Read the model definition and answer for the solid it produces. Units are mm, in the model's axes. Round coordinates to 2 decimals unless told otherwise and drop trailing zeros. Order: outer loops, then holes, each group sorted by start corner. A loop starts at its lowest first (then second) coordinate and runs counter-clockwise, first axis right, second up. Notation, with made-up numbers: (-20.75, -39.5) - (34.25, -39.5) arc R19 ccw to (34.25, -14.5) - close; hole circle Ø8 at (-32.75, -28). An arc over 180 degrees is marked (long way). Put each result on its own line as item: value. Start each with the question number.
Q1. Section A-A on x = 0 is taken. Give the vertices of the cut face in (y, z), then the cut area to 3 significant figures.
Q2. Find the intervals of material crossed by line 1 along Y through (x, z) = (1.5, 16.5); line 2 along Y through (x, z) = (-4.5, -22); line 3 along X through (y, z) = (39.5, 19.5), in increasing order. Write a range as from..to.
Q3. Section B-B on z = 0 is taken. Give the vertices of the cut face in (x, y), then the cut area to 3 significant figures.
Q4. Each of these flat-tipped pins is pushed along its axis until it touches: pin 1 Ø10 at (x, y) = (18, 29) entering from -Z; pin 2 Ø1 at (x, y) = (12.5, 50) entering from -Z; pin 3 Ø3 at (y, z) = (28.5, 9.5) entering from +X. Where does it stop, or does it pass through?
Q5. Section C-C on y = 14.5 is taken. Give the vertices of the cut face in (x, z).
Q6. For a pull along Y with two mould halves and no side action, classify faces 1 (the face through (4.01, 54.34, -18.04)), 2 (the face through (0, 0, 0)), 3 (the face through (14.59, 66.04, -11.19)), 4 (the face through (0, 71, 0)) as pulls with the +Y half, pulls with the -Y half, needs draft (parallel to the pull), parting line crosses it, or undercut.
Q7. Section D-D on y = 59 is taken. Give the vertices of the cut face in (x, z), then the cut area to 3 significant figures.
from build123d import *

# Parameters (mm, degrees)
SKETCH1_R           = 25.05
BOSS_EXTRUDE1_DEPTH = 71


with BuildPart() as part:
    # Sketch1 → Boss-Extrude1 (new body)
    with BuildSketch(Plane(origin=(0, 0, 0), x_dir=(1, 0, 0), z_dir=(0, 1, 0))):
        Circle(SKETCH1_R)
    extrude(amount=BOSS_EXTRUDE1_DEPTH)

    # Sketch2 → Cut-Revolve1 (revolve, cut)
    with BuildSketch(Plane.XY):
        with BuildLine():
            Line((-25.05, 67.7), (-18.045116148, 65.953486299))
            ThreePointArc((-18.045116148, 65.953486299), (-13.55, 60.2), (-18.045116148, 54.446513701))
            Line((-18.045116148, 54.446513701), (-25.05, 52.7))
            Line((-25.05, 52.7), (-25.05, 67.7))
        make_face()
    revolve(axis=Axis((0, -3.55, 0), (0, 1, 0)), mode=Mode.SUBTRACT)


solid = part.part
Findings:
1. outline: (0, -25.05) - (52.7, -25.05) - (54.45, -18.05) arc R5.93 cw to (65.95, -18.05) - (67.7, -25.05) - (71, -25.05) - (71, 25.05) - (67.7, 25.05) - (65.95, 18.05) arc R5.93 cw to (54.45, 18.05) - (52.7, 25.05) - (0, 25.05) - close
1. area: 3,290 mm2
2. line 1: 0..55.03, 65.37..71
2. line 2: 0..53.35, 67.05..71
2. line 3: -15.72..15.72
3. outline: (-25.05, 0) - (25.05, 0) - (25.05, 52.7) - (18.05, 54.45) arc R5.93 cw to (18.05, 65.95) - (25.05, 67.7) - (25.05, 71) - (-25.05, 71) - (-25.05, 67.7) - (-18.05, 65.95) arc R5.93 cw to (-18.05, 54.45) - (-25.05, 52.7) - close
3. area: 3,290 mm2
4. pin 1: z = -21.41
4. pin 2: z = -21.99
4. pin 3: x = 23.74
5. outline: circle Ø50.1 at (0, 0)
6. face 1: undercut
6. face 2: pulls with the -Y half
6. face 3: undercut
6. face 4: pulls with the +Y half
7. outline: circle Ø27.35 at (0, 0)
7. area: 587 mm2
